Can you work these out from the model? Positions are in its coordinate system, mm. Give positions to 0.01 mm unless a question says otherwise; leave off trailing zeros. Write each loop counter-clockwise with the first axis right and the second up, starting at its lowest first coordinate (ties: lowest second). Pieces come first, ordered by that corner, then holes. Notation, with made-up numbers: (-37.5, -12) -> (14.5, -12) arc R21 ccw to (14.5, -6) -> close; hole circle Ø11 at (-2.5, -9.75). An arc over 180 degrees is marked (long way). Answer as CSV lines item,"result". Start each with the question number.
1. If we section it at A-A on z = 181.5: Write out the boundary of the cut face in (x, y), plus the area to 3 significant figures.
2. I'm going to push flat-ended pins straight in: P1, Ø3.5, axis at x = 44.95, z = 47.48, coming from the +Y side; P2, Ø1.5, axis at x = 401.5, y = 1.5, coming from the +Z side. Where does each tip first touch, or does it pass through?
3. I need wall thicknesses on line 1 (X direction, y = 3.5, z = 175.47); line 2 (Z direction, x = 276.07, y = 1.3); line 3 (Z direction, x = 431.86, y = 3.65). Which ranges of each line are inside material? Lowest first, please. Write a range as [from, to].
```python
from build123d import *

# Parameters (mm, degrees)
BOSS_EXTRUDE1_DEPTH            = 5
M3_CLEARANCE_HOLE1_D           = 3.4
M3_CLEARANCE_HOLE1_CSINK_D     = 3.45
M3_CLEARANCE_HOLE1_CSINK_ANGLE = 90
M4_CLEARANCE_HOLE1_D           = 4.5
M4_CLEARANCE_HOLE1_CSINK_D     = 4.55
M4_CLEARANCE_HOLE1_CSINK_ANGLE = 90
M5_CLEARANCE_HOLE1_D           = 5.5
M5_CLEARANCE_HOLE1_CSINK_D     = 5.55
M5_CLEARANCE_HOLE1_CSINK_ANGLE = 90
M4_CLEARANCE_HOLE2_D           = 4.5
M4_CLEARANCE_HOLE2_CSINK_D     = 4.55
M4_CLEARANCE_HOLE2_CSINK_ANGLE = 90


with BuildPart() as part:
    # Sketch1 → Boss-Extrude1 (new body)
    with BuildSketch(Plane(origin=(0, 0, 0), x_dir=(1, 0, 0), z_dir=(0, 1, 0))):
        Polygon((0, 0), (0, -220), (300, -220), (300, -170), (450, -170), (450, 0), align=None)
    extrude(amount=BOSS_EXTRUDE1_DEPTH)

    # M3 Clearance Hole1 (through all)
    with Locations(Plane(origin=(0, 5, 0), x_dir=(1, 0, 0), z_dir=(0, 1, 0))):
        with Locations((17.79, -175.47), (45.79, -197.97), (84.79, -175.47), (251.48, -204.04), (251.48, -165.94), (149.84, -139.45), (217.84, -85.45), (149.84, -31.45), (289.58, -165.94), (289.58, -204.04)):
            CounterSinkHole(M3_CLEARANCE_HOLE1_D / 2, M3_CLEARANCE_HOLE1_CSINK_D / 2, counter_sink_angle=M3_CLEARANCE_HOLE1_CSINK_ANGLE)

    # M4 Clearance Hole1 (through all)
    with Locations(Plane(origin=(0, 5, 0), x_dir=(1, 0, 0), z_dir=(0, 1, 0))):
        with Locations((44.95, -47.48), (89.15, -47.48), (67.05, -127.48), (276.07, -29.99), (325.07, -29.99), (276.07, -136.99), (325.07, -136.99), (225, -199.19), (225, -169.19), (110.5, -191), (196.5, -191)):
            CounterSinkHole(M4_CLEARANCE_HOLE1_D / 2, M4_CLEARANCE_HOLE1_CSINK_D / 2, counter_sink_angle=M4_CLEARANCE_HOLE1_CSINK_ANGLE)

    # M5 Clearance Hole1 (through all)
    with Locations(Plane(origin=(431.86, 5, 50.98), x_dir=(0, 0, 1), z_dir=(0, 1, 0))):
        with Locations((0, 0), (60, 0)):
            CounterSinkHole(M5_CLEARANCE_HOLE1_D / 2, M5_CLEARANCE_HOLE1_CSINK_D / 2, counter_sink_angle=M5_CLEARANCE_HOLE1_CSINK_ANGLE)

    # M4 Clearance Hole2 (through all)
    with Locations(Plane(origin=(0, 5, 0), x_dir=(1, 0, 0), z_dir=(0, 1, 0))):
        with Locations((76, -8), (76, -163), (76, -211), (374, -151), (374, -16)):
            CounterSinkHole(M4_CLEARANCE_HOLE2_D / 2, M4_CLEARANCE_HOLE2_CSINK_D / 2, counter_sink_angle=M4_CLEARANCE_HOLE2_CSINK_ANGLE)


solid = part.part
```
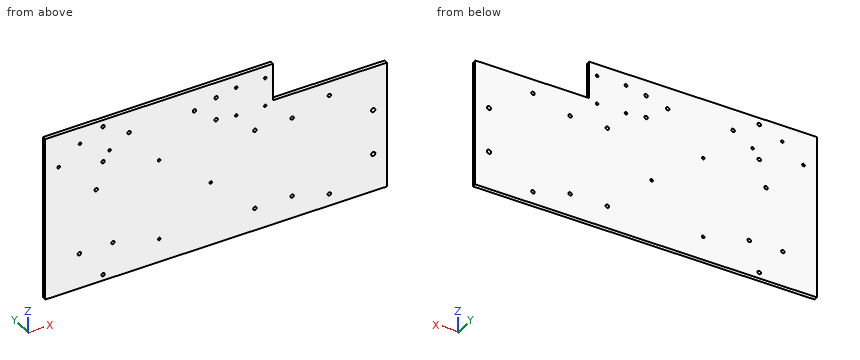
Computed values:
1,outline,"(0, 0) -> (300, 0) -> (300, 5) -> (0, 5) -> close"
1,area,"1,500 mm2"
2,P1,"passes through"
2,P2,"stops at z = 170"
3,line 1,"x = [0, 16.09], [19.49, 83.09], [86.49, 300]"
3,line 2,"z = [0, 27.74], [32.24, 134.74], [139.24, 220]"
3,line 3,"z = [0, 48.23], [53.73, 108.23], [113.73, 170]"
